For this review, take the finished solid that the model builds, in its own axes (mm). Round coordinates to 2 decimals unless told otherwise and drop trailing zeros.
from build123d import *

# Parameters (mm, degrees)
F0_W     = 149.86
F0_H     = 50.8
F1_DEPTH = 4.064
F3_D     = 4.572


with BuildPart() as f1:
    # F0 (on Top) → F1 (new body)
    with BuildSketch(Plane.XY):
        Rectangle(F0_W, F0_H)
    extrude(amount=F1_DEPTH)

    # F3 (through all)
    with Locations(Plane.XY.offset(4.064)):
        with Locations((-62.738, 13.208), (-25.908, 13.208), (-25.908, -13.208), (-62.738, -13.208), (25.908, 13.208), (62.738, 13.208), (62.738, -13.208), (25.908, -13.208)):
            Hole(F3_D / 2)


solid = f1.part
(1) For line 1 along X through (y, z) = (-11.5, 0.6); line 2 along Y through (x, z) = (-24.5, 0.5); line 3 along X through (y, z) = (13, 0.4), list the stretches that pass through material, from the lowest coordinate up.
Geometry check:
line 1: x = -74.93 to -64.26, -61.22 to -27.43, -24.39 to 24.39, 27.43 to 61.22, 64.26 to 74.93
line 2: y = -25.4 to -15.01, -11.41 to 11.41, 15.01 to 25.4
line 3: x = -74.93 to -65.01, -60.46 to -28.18, -23.63 to 23.63, 28.18 to 60.46, 65.01 to 74.93
(2) Mouldability with a two-part tool opening along Y and no side actions: class faces 1 (the face through (-1, -25.4, 2)), 2 (the face through (28.19, 13.31, 2)), 3 (the face through (-1, 0, 0)) as pulls with the +Y half, pulls with the -Y half, needs draft (parallel to the pull), parting line crosses it, or undercut.
Geometry check:
face 1: pulls with the -Y half
face 2: undercut
face 3: needs draft
(3) We need section A-A, the plane z = 3.35. State how many separate pieces and enclosed holes the cut face has, and give its area (3 significant figures).
Geometry check:
separate pieces: 1
enclosed holes: 8
area: 7,480 mm2
